from build123d import *

# Parameters (mm, degrees)
F0_W        = 60
F0_H        = 1.5
F1_DEPTH    = 20
F2_W        = 10.4806274176
F2_H        = 3.8417847827
F3_DEPTH    = 2.54
F4_T1_DEPTH = 7.7522870812


# Not quite as in the source:
# - a fillet or chamfer that OpenCascade refuses, or shapes differently, is made with other operations: its cross-section is extruded or revolved along the edge and cut away or added


with BuildPart() as f1:
    # F0 (on Front) → F1 (new body, symmetric)
    with BuildSketch(Plane.XZ):
        Rectangle(F0_W, F0_H)
    extrude(amount=F1_DEPTH, both=True)

    # F2 (on face) → F3 (join)
    with BuildSketch(Plane.XY.offset(0.75)):
        with Locations((-22.3847124726, 17.5385358743)):
            Rectangle(F2_W, F2_H)
    extrude(amount=F3_DEPTH)

    # F4: fillet of radius 2.0849148325 on 4 edges, made by hand

    # F4_s2 → F4_t1 (cut)
    with BuildSketch(Plane.XY.offset(0.75)):
        with BuildLine():
            ThreePointArc((-27.6250261813, 17.7025583154), (-27.0143687651, 16.2283008992), (-25.5401113489, 15.617643483))
            Line((-25.5401113489, 15.617643483), (-27.6250261813, 15.617643483))
            Line((-27.6250261813, 15.617643483), (-27.6250261813, 17.7025583154))
        make_face()
        with BuildLine():
            ThreePointArc((-25.5401113489, 19.4594282657), (-27.0143687651, 18.8487708495), (-27.6250261813, 17.3745134332))
            Line((-27.6250261813, 17.3745134332), (-27.6250261813, 19.4594282657))
            Line((-27.6250261813, 19.4594282657), (-25.5401113489, 19.4594282657))
        make_face()
        with BuildLine():
            ThreePointArc((-19.2293135962, 15.617643483), (-17.75505618, 16.2283008992), (-17.1443987638, 17.7025583154))
            Line((-17.1443987638, 17.7025583154), (-17.1443987638, 15.617643483))
            Line((-17.1443987638, 15.617643483), (-19.2293135962, 15.617643483))
        make_face()
        with BuildLine():
            ThreePointArc((-19.2293135962, 19.4594282657), (-17.75505618, 18.8487708495), (-17.1443987638, 17.3745134332))
            Line((-17.1443987638, 17.3745134332), (-17.1443987638, 19.4594282657))
            Line((-17.1443987638, 19.4594282657), (-19.2293135962, 19.4594282657))
        make_face()
    extrude(amount=F4_T1_DEPTH, mode=Mode.SUBTRACT)


solid = f1.part
Read the model definition and answer for the solid it produces. Units are mm, in the model's axes. A direction names the side the tool comes from. Coordinates: 2 decimals unless noted, no trailing zeros. Loops run counter-clockwise (first coordinate to the right, second up) from the corner with the lowest first, then second, coordinate; pieces in that order, holes last. Notation, with made-up numbers: (62.5, 80) -> (98.5, 80) arc R20 ccw to (98.5, 88) -> close; hole circle Ø3 at (-18.5, 88.5). An arc over 180 degrees is marked (long way). Write item = value, one per line. Start each with the question number.
1) For faces 1 (the face through (-17.83, 16.157, 2.002)), 2 (the face through (-17.83, 18.92, 2)), 3 (the face through (-26.94, 18.92, 2)), 4 (the face through (-22, 15.618, 2)), determine the directions among +Z, -Z, +X, -X, +Y, -Y from which every point of the face is accessible in a straight line to the end or side of a thin tool.
2) Find the intervals of material crossed by L1, parallel to Z at x = -9.5, y = 14.5; L2, parallel to Y at x = -19.5, z = 2.95; L3, parallel to X at y = 16, z = 1.95, in increasing order. Write a range as from..to.
3) The part is cut by section B-B, the plane z = 2.45. Determine the outline of the cut face in (x, y).
4) The part is cut by section A-A, the plane x = -24.5. Determine the outline of the cut face in (y, z), plus the area to 3 significant figures.
5) Given P1, Ø12, axis at x = -9, y = 1.5, coming from the +Z side; P2, Ø1.5, axis at x = -14, z = 2.5, coming from the -Y side; P3, Ø1.3, axis at x = -23, z = 2.5, coming from the -Y side, each flat-ended and moving along its own axis, determine where each tip first touches the part or whether it passes through.
6) The part is cut by section D-D, the plane x = 13. Determine the outline of the cut face in (y, z).
7) The part is cut by section C-C, the plane y = -10.5. Determine the outline of the cut face in (x, z), plus the area to 3 significant figures.
Result:
q1.face_1 = +Z, +X, -Y
q1.face_2 = +Z, +X, +Y
q1.face_3 = +Z, -X, +Y
q1.face_4 = +Z, +X, -X, -Y
q2.L1 = -0.75..0.75
q2.L2 = 15.62..19.46
q2.L3 = -26.74..-18.03
q3.outline = (-27.62, 17.54) arc R2.08 ccw to (-25.54, 15.62) -> (-19.23, 15.62) arc R2.08 ccw to (-17.15, 17.54) arc R2.08 ccw to (-19.23, 19.46) -> (-25.54, 19.46) arc R2.08 ccw to start
q4.outline = (-20, -0.75) -> (20, -0.75) -> (20, 0.75) -> (19.46, 0.75) -> (19.46, 3.29) -> (15.62, 3.29) -> (15.62, 0.75) -> (-20, 0.75) -> close
q4.area = 69.8 mm²
q5.P1 = 0.75
q5.P2 = through
q5.P3 = 15.62
q6.outline = (-20, -0.75) -> (20, -0.75) -> (20, 0.75) -> (-20, 0.75) -> close
q7.outline = (-30, -0.75) -> (30, -0.75) -> (30, 0.75) -> (-30, 0.75) -> close
q7.area = 90.0 mm²
